```python
from build123d import *

# Parameters (mm, degrees)
F0_W     = 500
F0_H     = 500
F0_R     = 118.0247003556
F0_W_2   = 75
F0_H_2   = 75
F1_DEPTH = 50
F2_DEPTH = 40
F3_R     = 7.5


with BuildPart() as f1:
    # F0 (on Top) → F1 (new body)
    with BuildSketch(Plane.XY):
        Rectangle(F0_W, F0_H)
        Polygon((-191.2311762839, 43.6472680867), (-85.1058798965, 176.7241805792), (85.1058798965, 176.7241805792), (191.2311762839, 43.6472680867), (153.3554965244, -122.296927517), (0, -196.1490422978), (-153.3554965244, -122.296927517), align=None, mode=Mode.SUBTRACT)
        Polygon((85.1058798965, 176.7241805792), (-85.1058798965, 176.7241805792), (-191.2311762839, 43.6472680867), (-153.3554965244, -122.296927517), (0, -196.1490422978), (153.3554965244, -122.296927517), (191.2311762839, 43.6472680867), align=None)
        Circle(F0_R, mode=Mode.SUBTRACT)
        Circle(F0_R)
        Rectangle(F0_W_2, F0_H_2, mode=Mode.SUBTRACT)
        Rectangle(F0_W_2, F0_H_2)
    extrude(amount=F1_DEPTH)

    # F0 (on Top) → F2 (cut)
    with BuildSketch(Plane.XY):
        Polygon((85.1058798965, 176.7241805792), (-85.1058798965, 176.7241805792), (-191.2311762839, 43.6472680867), (-153.3554965244, -122.296927517), (0, -196.1490422978), (153.3554965244, -122.296927517), (191.2311762839, 43.6472680867), align=None)
        Circle(F0_R, mode=Mode.SUBTRACT)
        Rectangle(F0_W_2, F0_H_2)
    extrude(amount=F2_DEPTH, mode=Mode.SUBTRACT)

    # F3
    f3_edges = [f1.edges().sort_by_distance(p)[0] for p in [
        (250, -250, 25),
        (-250, -250, 25),
        (-250, 250, 25),
        (250, 250, 25),
        (0, -196.149042, 20),
        (-153.355497, -122.296928, 20),
        (153.355497, -122.296928, 20),
        (191.231176, 43.647268, 20),
        (85.10588, 176.724181, 20),
        (-85.10588, 176.724181, 20),
        (-191.231176, 43.647268, 20),
        (-37.5, -37.5, 20),
        (37.5, -37.5, 20),
        (37.5, 37.5, 20),
        (-37.5, 37.5, 20),
    ]]
    fillet(f3_edges, radius=F3_R)


solid = f1.part
```
Geometry: final body of the model. Coordinates: model frame, mm. A direction names the side the tool comes from. Round coordinates to 2 decimals unless told otherwise and drop trailing zeros. Write each loop counter-clockwise with the first axis right and the second up, starting at its lowest first coordinate (ties: lowest second). Pieces come first, ordered by that corner, then holes. Notation, with made-up numbers: (-20.5, 44) -> (12.5, 44) arc R22 cw to (12.5, 52) -> close; hole circle Ø2 at (-32.75, 31). An arc over 180 degrees is marked (long way). Return JSON: item names as keys, results as strings.
Q1. Set-up query: faces 4 (the flat face through (-137.457, 111.078, 19.72)), 5 (the flat face through (-3, 250, 25)). Return all of +Z, -Z, +X, -X, +Y, -Y with unobstructed straight access to the full face (end or side cutting, diameter ignored); none if empty.
From the geometry:
{"face 4": "-Z", "face 5": "+Z, -Z, +X, -X, +Y"}
Q2. Section C-C on y = 0. Return the cut outline in (x, z), and give its area (3 significant figures).
From the geometry:
{"outline": "(-250, 0) -> (-181.27, 0) -> (-181.27, 40) -> (-118.02, 40) -> (-118.02, 0) -> (-37.5, 0) -> (-37.5, 40) -> (37.5, 40) -> (37.5, 0) -> (118.02, 0) -> (118.02, 40) -> (181.27, 40) -> (181.27, 0) -> (250, 0) -> (250, 50) -> (-250, 50) -> close", "area": "16,900 mm2"}
Q3. Section B-B on y = 140.5. Return the cut outline in (x, z).
From the geometry:
{"outline": "(-250, 0) -> (-113.99, 0) -> (-113.99, 40) -> (113.99, 40) -> (113.99, 0) -> (250, 0) -> (250, 50) -> (-250, 50) -> close"}
Q4. Ray query, line 1 (Y direction, x = 88.5, z = 28.5); line 2 (X direction, y = -55.5, z = 17.5); line 3 (X direction, y = 67.5, z = 26). Return the intervals inside material, ascending.
From the geometry:
{"line 1": "-250 to -153.53, -78.09 to 78.09, 172.47 to 250", "line 2": "-250 to -168.6, -104.16 to 104.16, 168.6 to 250", "line 3": "-250 to -172.21, -96.82 to 96.82, 172.21 to 250"}
Q5. Mould query, pull axis Y, two halves, no side actions, for faces 1 (the flat face through (82, -89, 40)), 2 (the flat face through (-3, 4, 50)), 3 (the flat face through (-3, -250, 25)). Classes: +Y half, -Y half, draft (parallel to the pull), parting line (faces both ways), or undercut.
From the geometry:
{"face 1": "undercut", "face 2": "draft", "face 3": "-Y half"}
Q6. First-contact query: pin 1 Ø1.5 at (x, y) = (116.5, -109.5) entering from -Z. Flat tip, straight axial feed; report the tip coordinate or a pass-through.
From the geometry:
{"pin 1": "z = 40"}
Q7. Section A-A on x = 169. Return the cut outline in (y, z).
From the geometry:
{"outline": "(-250, 0) -> (-53.75, 0) -> (-53.75, 40) -> (71.52, 40) -> (71.52, 0) -> (250, 0) -> (250, 50) -> (-250, 50) -> close"}
